Here's how the part is built. I have some questions about the finished solid (model axes, mm). A direction names the side the tool comes from. Coordinates: 2 decimals unless noted, no trailing zeros. Loops run counter-clockwise (first coordinate to the right, second up) from the corner with the lowest first, then second, coordinate; pieces in that order, holes last. Notation, with made-up numbers: (50.25, -14) -> (96.25, -14) arc R9 cw to (96.25, 2) -> close; hole circle Ø7 at (67.5, -4). An arc over 180 degrees is marked (long way). Answer as a JSON object with one key per item and string values. Group by question number.
Q1. I want a section at A-A on y = 0. Write out the boundary of the cut face in (x, z), then the cut area to 3 significant figures.
Q2. I'm going to push flat-ended pins straight in: pin 1 (5 mm diameter, centred on y = -5, z = 10, fed in from +X); pin 2 (1 mm diameter, centred on x = 32.5, z = 2.5, fed in from -Y); pin 3 (8 mm diameter, centred on y = 15, z = 6, fed in from +X) (3 decimals). Where does each tip first touch, or does it pass through?
Q3. Thinking about a two-plate mould opening in X: for faces 1 (the flat face through (9.4, 18.3, -15)), 2 (the cylindrical face through (47.69, 15.02, 0.28)), 3 (the cylindrical face through (-8.67, -39.05, 17.54)), 4 (the flat face through (-22, 34, 20)), which applies, released by +X, released by -X, zero draft, split by the parting line, or undercut?
Q4. On a 3-axis mill with a long thin cutter (end or side, diameter ignored), from which of +Z, -Z, +X, -X, +Y, -Y can I reach the whole of each face in a straight line? I mean faces 5 (the cylindrical face through (4.336, 19.524, -17.465)), 6 (the flat face through (-5, 9, 20)), 7 (the flat face through (-9.4, 18.3, 15)). Say none if no direction works.
Q5. I want a section at C-C on z = -16.5. Write out the boundary of the cut face in (x, y).
Q6. I want a section at D-D on z = -8. Write out the boundary of the cut face in (x, y), then the cut area to 3 significant figures.
Q7. I need wall thicknesses on line 1 (Y direction, x = 0, z = 17.5); line 2 (Y direction, x = 0, z = -3); line 3 (Z direction, x = -25, y = 22). Which ranges of each line are inside material? Lowest first, please.
Autodesk Inventor part; units mm, degrees
ref_plane "YZ Plane" through (0, 0, 0) normal (1, 0, 0) x (0, 1, 0)
ref_plane "XZ Plane" through (0, 0, 0) normal (0, 1, 0) x (-1, 0, 0)
ref_plane "XY Plane" through (0, 0, 0) normal (0, 0, 1) x (1, 0, 0)
sketch "Esboço1" plane through (0, 0, 0) normal (0, 0, 1) x (1, 0, 0)
  circle A0 centre (0, 0) radius 10
  circle A1 centre (0, 0) radius 40
  circle A2 centre (0, 0) radius 50
  dimension "d0" = 100
  dimension "d1" = 80
  dimension "d2" = 20
extrude "Extrusão1" add sketch "Esboço1" along normal mid plane 40 contours A1 | A2
sketch "Esboço2" plane through (0, 0, 20) normal (0, 0, 1) x (1, 0, 0)
  circle A0 centre (0, 0) radius 40
  dimension "d5" = 80
extrude "Extrusão2" cut sketch "Esboço2" against normal blind 5
sketch "Esboço3" plane through (0, 0, -20) normal (0, 0, -1) x (-1, 0, 0)
  circle A0 centre (0, 0) radius 40
  dimension "d8" = 80
extrude "Extrusão3" cut sketch "Esboço3" against normal blind 5
sketch "Esboço4" plane through (0, 0, 15) normal (0, 0, 1) x (1, 0, 0)
  circle A0 centre (0, 0) radius 20
  dimension "d11" = 40
extrude "Extrusão4" add sketch "Esboço4" along normal blind 5
sketch "Esboço5" plane through (0, 0, -15) normal (0, 0, -1) x (-1, 0, 0)
  circle A0 centre (0, 0) radius 20
  dimension "d14" = 40
extrude "Extrusão5" add sketch "Esboço5" along normal blind 5
sketch "Esboço6" plane through (0, 0, 20) normal (0, 0, 1) x (1, 0, 0)
  circle A0 centre (0, 0) radius 10
  dimension "d17" = 20
extrude "Extrusão6" cut sketch "Esboço6" against normal through all
properties part number "rodizio"
Result set:
{
 "1": {"outline": "(-50, -20) -> (-40, -20) -> (-40, -15) -> (-20, -15) -> (-20, -20) -> (-10, -20) -> (-10, 20) -> (-20, 20) -> (-20, 15) -> (-40, 15) -> (-40, 20) -> (-50, 20) -> close; (10, -20) -> (20, -20) -> (20, -15) -> (40, -15) -> (40, -20) -> (50, -20) -> (50, 20) -> (40, 20) -> (40, 15) -> (20, 15) -> (20, 20) -> (10, 20) -> close", "area": "2,800 mm²"},
 "2": {"pin 1": "stops at x = 49.94", "pin 2": "stops at y = -38.42", "pin 3": "stops at x = 48.775"},
 "3": {"face 1": "undercut", "face 2": "split by the parting line", "face 3": "undercut", "face 4": "zero draft"},
 "4": {"face 5": "-Z", "face 6": "+Z, +X, -X, +Y, -Y", "face 7": "+Z"},
 "5": {"outline": "circle Ø100 at (0, 0); circle Ø40 at (0, 0); hole circle Ø80 at (0, 0); hole circle Ø20 at (0, 0)"},
 "6": {"outline": "circle Ø100 at (0, 0); hole circle Ø20 at (0, 0)", "area": "7,540 mm²"},
 "7": {"line 1": "y = -50 to -40, -20 to -10, 10 to 20, 40 to 50", "line 2": "y = -50 to -10, 10 to 50", "line 3": "z = -15 to 15"}
}
